Design review of the part built by this model. Coordinates are the model's own, in mm. A direction names the side the tool comes from. Coordinates: 2 decimals unless noted, no trailing zeros. Write each loop counter-clockwise with the first axis right and the second up, starting at its lowest first coordinate (ties: lowest second). Pieces come first, ordered by that corner, then holes.
Q1. Take a section at A-A (y = 52.5). Give the boundary of the cut face in (x, z) (3 decimals), and give its area (3 significant figures).
Q2. Take a section at B-B (z = 11.5). Give the boundary of the cut face in (x, y).
Q3. Take a section at C-C (x = 3.5). Give the boundary of the cut face in (y, z) (3 decimals).
Q4. Take a section at D-D (x = 73.5). Give the boundary of the cut face in (y, z), and give its area (4 significant figures).
Q5. Insertion check: pin 1 (2 mm diameter, centred on y = 25, z = 11, fed in from -X); pin 2 (6 mm diameter, centred on x = 70.5, y = 26.5, fed in from -Z); pin 3 (7 mm diameter, centred on y = 10, z = 10, fed in from -X); pin 4 (5 mm diameter, centred on x = 78.5, z = 12, fed in from +Y). Each pin has a flat end and moves straight along its axis. Give the tip position at first contact, or say it passes through.
Q6. Machinability: for faces 4 (the flat face through (76, 10, 15)), 5 (the flat face through (66.5, 10, 8)), 6 (the flat face through (68.5, 47, 9)), 7 (the cylindrical face through (4.77, 2.97, 0.74)), 8 (the flat face through (76, 17.75, 8)), which of the approach directions +Z, -Z, +X, -X, +Y, -Y give a long, thin tool a straight path to every point of the face, cutting with its end or side? Answer none if there is none.
Q7. For probe 1 along Y at (x, z) = (3.5, 0.9) (3 decimals); probe 2 along Y at (x, z) = (83, 13); probe 3 along X at (y, z) = (34, 12.5), list the stretches that pass through material, from the lowest coordinate up.
Q8. Mouldability with a two-part tool opening along Y and no side actions: class faces 1 (the cylindrical face through (62.77, 2.97, 0.74)), 2 (the flat face through (77, 53.5, 9)), 3 (the flat face through (68.5, 29, 9)) as pulls with the +Y half, pulls with the -Y half, needs draft (parallel to the pull), parting line crosses it, or undercut.
```python
from build123d import *

# Parameters (mm, degrees)
F0_W     = 85
F0_H     = 56
F0_R     = 1.375
F1_DEPTH = 1.5
F3_W     = 18
F3_H     = 13
F4_DEPTH = 16
F3_W_2   = 20
F3_H_2   = 15
F5_DEPTH = 13.5


# Not quite as in the source:
# - a feature names something its author has since deleted; it is built from what else it names


with BuildPart() as f1:
    # F0 (on Top) → F1 (new body)
    with BuildSketch(Plane.XY):
        with Locations((42.5, 28)):
            Rectangle(F0_W, F0_H)
        with Locations((3.5, 3.5)):
            Circle(F0_R, mode=Mode.SUBTRACT)
        with Locations((61.5, 3.5)):
            Circle(F0_R, mode=Mode.SUBTRACT)
        with Locations((3.5, 52.5)):
            Circle(F0_R, mode=Mode.SUBTRACT)
        with Locations((61.5, 52.5)):
            Circle(F0_R, mode=Mode.SUBTRACT)
    extrude(amount=F1_DEPTH)

    # F3 (on offset) → F4 (join)
    with BuildSketch(Plane.XY.offset(1.5)):
        with Locations((77.5, 47)):
            Rectangle(F3_W, F3_H)
        with Locations((77.5, 29)):
            Rectangle(F3_W, F3_H)
    extrude(amount=F4_DEPTH)

    # F3 (on offset) → F5 (join)
    with BuildSketch(Plane.XY.offset(1.5)):
        with Locations((76.5, 10.25)):
            Rectangle(F3_W_2, F3_H_2)
    extrude(amount=F5_DEPTH)


solid = f1.part
```
Response:
1. outline: (0, 0) - (2.125, 0) - (2.125, 1.5) - (0, 1.5) - close; (4.875, 0) - (60.125, 0) - (60.125, 1.5) - (4.875, 1.5) - close; (62.875, 0) - (85, 0) - (85, 1.5) - (86.5, 1.5) - (86.5, 17.5) - (68.5, 17.5) - (68.5, 1.5) - (62.875, 1.5) - close
1. area: 407 mm2
2. outline: (66.5, 2.75) - (86.5, 2.75) - (86.5, 17.75) - (66.5, 17.75) - close; (68.5, 22.5) - (86.5, 22.5) - (86.5, 35.5) - (68.5, 35.5) - close; (68.5, 40.5) - (86.5, 40.5) - (86.5, 53.5) - (68.5, 53.5) - close
3. outline: (0, 0) - (2.125, 0) - (2.125, 1.5) - (0, 1.5) - close; (4.875, 0) - (51.125, 0) - (51.125, 1.5) - (4.875, 1.5) - close; (53.875, 0) - (56, 0) - (56, 1.5) - (53.875, 1.5) - close
4. outline: (0, 0) - (56, 0) - (56, 1.5) - (53.5, 1.5) - (53.5, 17.5) - (40.5, 17.5) - (40.5, 1.5) - (35.5, 1.5) - (35.5, 17.5) - (22.5, 17.5) - (22.5, 1.5) - (17.75, 1.5) - (17.75, 15) - (2.75, 15) - (2.75, 1.5) - (0, 1.5) - close
4. area: 702.5 mm2
5. pin 1: stops at x = 68.5
5. pin 2: stops at z = 0
5. pin 3: stops at x = 66.5
5. pin 4: stops at y = 53.5
6. face 4: +Z, +X, -X, -Y
6. face 5: +Z, -X, +Y, -Y
6. face 6: +Z, -X, +Y
6. face 7: +Z, -Z
6. face 8: +Z, +X, -X
7. probe 1: y = 0 to 2.125, 4.875 to 51.125, 53.875 to 56
7. probe 2: y = 2.75 to 17.75, 22.5 to 35.5, 40.5 to 53.5
7. probe 3: x = 68.5 to 86.5
8. face 1: undercut
8. face 2: pulls with the +Y half
8. face 3: needs draft
